Input: part model. Units: mm. Frame: model coordinates. Face numbers are marked on the shaded views. A direction names the side the tool comes from. Round coordinates to 2 decimals unless told otherwise and drop trailing zeros. Loops run counter-clockwise (first coordinate to the right, second up) from the corner with the lowest first, then second, coordinate; pieces in that order, holes last. Notation, with made-up numbers: (46, -17.75) -> (58, -17.75) arc R20 cw to (58, -1.75) -> close; hole circle Ø10 at (76, 47.25). An arc over 180 degrees is marked (long way). Answer as a JSON object with one key per item and string values.
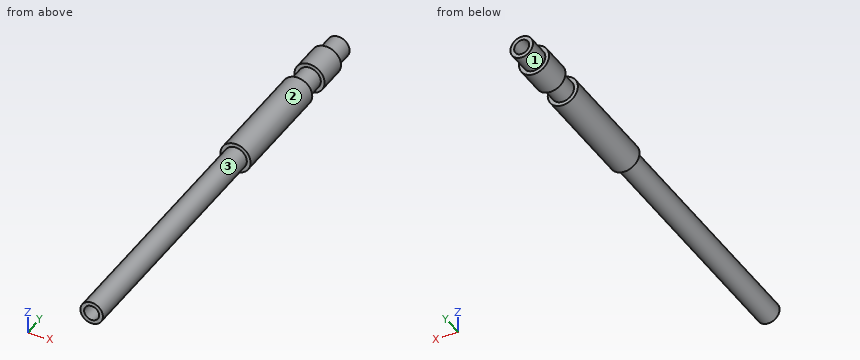
```python
from build123d import *

# Parameters (mm, degrees)
SKETCH_1_R      = 2
SKETCH_1_R_2    = 1
EXTRUDE_1_DEPTH = 60
SKETCH_2_W      = 0.5
SKETCH_2_H      = 3
SKETCH_3_W      = 0.5
SKETCH_3_H      = 35


with BuildPart() as part:
    # Эскиз1 → Бобышка-Вытянуть1 (new body)
    with BuildSketch(Plane(origin=(0, 0, 0), x_dir=(1, 0, 0), z_dir=(0, 1, 0))):
        Circle(SKETCH_1_R)
        Circle(SKETCH_1_R_2, mode=Mode.SUBTRACT)
    extrude(amount=EXTRUDE_1_DEPTH)

    # Эскиз2 → Вырез-Повернуть1 (revolve, cut)
    with BuildSketch(Plane.XY):
        with Locations((1.75, 58.5)):
            Rectangle(SKETCH_2_W, SKETCH_2_H)
        with Locations((1.75, 51.5)):
            Rectangle(SKETCH_2_W, SKETCH_2_H)
    revolve(axis=Axis((0, 60, 0), (0, -1, 0)), mode=Mode.SUBTRACT)

    # Эскиз3 → Вырез-Повернуть2 (revolve, cut)
    with BuildSketch(Plane.XY):
        with Locations((1.75, 17.5)):
            Rectangle(SKETCH_3_W, SKETCH_3_H)
    revolve(axis=Axis((0, 0, 0), (0, 1, 0)), mode=Mode.SUBTRACT)


solid = part.part
```
1) Ray query, probe 1 along Y at (x, z) = (1.7, -0.15); probe 2 along X at (y, z) = (32, 0). Return the intervals inside material, ascending.
Output:
{"probe 1": "y = 35 to 50, 53 to 57", "probe 2": "x = -1.5 to -1, 1 to 1.5"}
2) Reachability of the marked faces 1, 2 and 3 from +Z, -Z, +X, -X, +Y, -Y: full face, straight path, thin tool, end or side. Return the list, or none.
Output:
{"face 1": "+Y", "face 2": "+Y, -Y", "face 3": "-Y"}
3) Contact query for flat-ended pins moving along their axis: P1, Ø2, axis at y = 26.5, z = -1.5, coming from the +X side; P2, Ø1.5, axis at y = 30.5, z = -1.5, coming from the +X side; P3, Ø1.5, axis at y = 19, z = -1, coming from the -X side. Output: stop coordinate, or through.
Output:
{"P1": "stops at x = 1.41", "P2": "stops at x = 1.3", "P3": "stops at x = -1.48"}
4) Section A-A, the plane x = 0. Output: boundary loops of the cut face in (y, z), plus the area to 3 significant figures.
Output:
{"outline": "(0, -1.5) -> (35, -1.5) -> (35, -2) -> (50, -2) -> (50, -1.5) -> (53, -1.5) -> (53, -2) -> (57, -2) -> (57, -1.5) -> (60, -1.5) -> (60, -1) -> (0, -1) -> close; (0, 1) -> (60, 1) -> (60, 1.5) -> (57, 1.5) -> (57, 2) -> (53, 2) -> (53, 1.5) -> (50, 1.5) -> (50, 2) -> (35, 2) -> (35, 1.5) -> (0, 1.5) -> close", "area": "79.0 mm^2"}
5) Section C-C, the plane y = 24. Output: boundary loops of the cut face in (x, z).
Output:
{"outline": "circle Ø3 at (0, 0); hole circle Ø2 at (0, 0)"}
6) Section B-B, the plane z = 0. Output: boundary loops of the cut face in (x, y), plus the area to 3 significant figures.
Output:
{"outline": "(-2, 35) -> (-1.5, 35) -> (-1.5, 0) -> (-1, 0) -> (-1, 60) -> (-1.5, 60) -> (-1.5, 57) -> (-2, 57) -> (-2, 53) -> (-1.5, 53) -> (-1.5, 50) -> (-2, 50) -> close; (1, 0) -> (1.5, 0) -> (1.5, 35) -> (2, 35) -> (2, 50) -> (1.5, 50) -> (1.5, 53) -> (2, 53) -> (2, 57) -> (1.5, 57) -> (1.5, 60) -> (1, 60) -> close", "area": "79.0 mm^2"}
